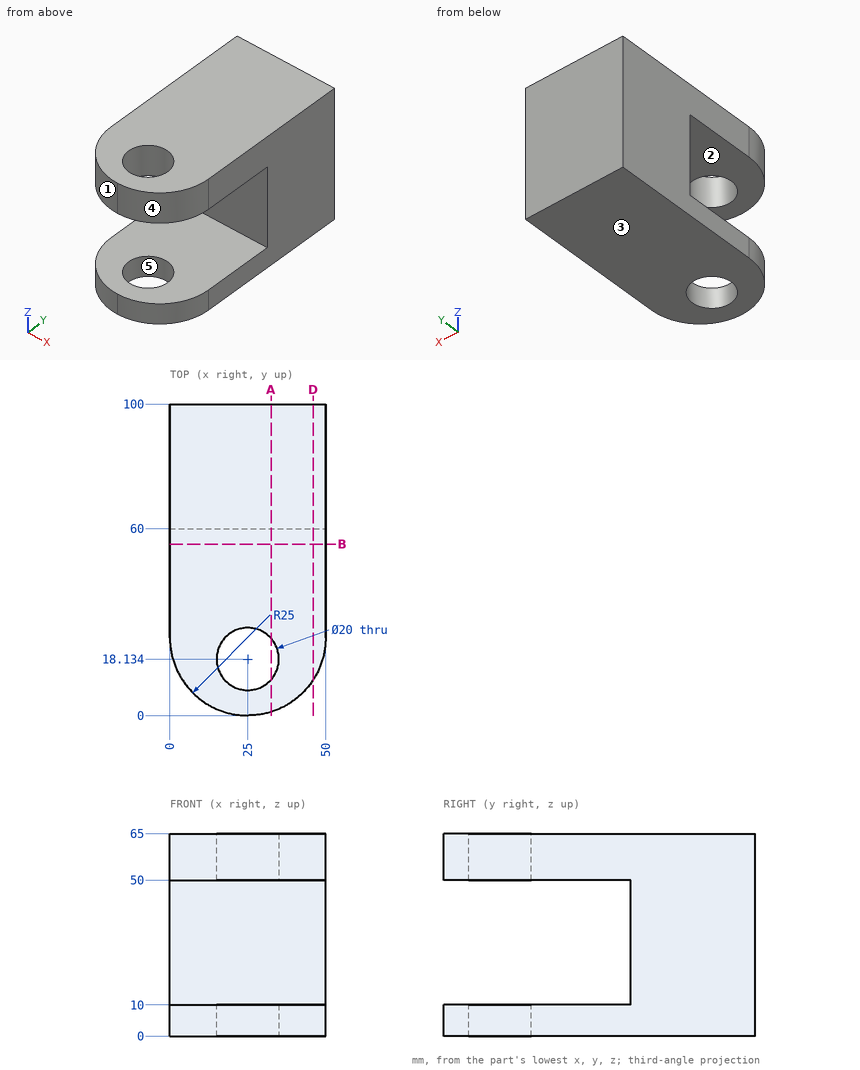
Source: three-view drawing plus pictorial views. Frame: mm from the lowest corner of the part. A direction names the side the tool comes from. Give positions to 0.01 mm unless a question says otherwise; leave off trailing zeros. Loops run counter-clockwise (first coordinate to the right, second up) from the corner with the lowest first, then second, coordinate; pieces in that order, holes last. Notation, with made-up numbers: (42, 21.25) -> (54, 21.25) arc R17 cw to (54, 30.25) -> close; hole circle Ø3 at (-8.75, -26.75). An arc over 180 degrees is marked (long way). Put each result on its own line as item: value. Start each with the question number.
1) Cut plane D-D (x = 46). Return loops of the section in (y, z) (1 decimal).
2) Contact query for flat-ended pins moving along their axis: P1, Ø5, axis at y = 16.5, z = 53, coming from the +X side; P2, Ø12, axis at x = 17, z = 21.5, coming from the -Y side. Output: stop coordinate, or through.
3) Cut plane A-A (x = 32.5). Return loops of the section in (y, z), then the cut area to 3 significant figures.
4) Cut plane B-B (y = 55). Return loops of the section in (x, z).
5) Draft query along Y for the marked faces 3, 4 and 5. Return one class per face: released by +Y, released by -Y, zero draft, split by the parting line, or undercut.
6) Material intervals for probe 1 along Z at (x, y) = (20.5, 59); probe 2 along Y at (x, z) = (25, 4); probe 3 along Y at (x, z) = (33.5, 18.5), sorted ascending.
7) Reachability of the marked faces 1 and 2 from +Z, -Z, +X, -X, +Y, -Y: full face, straight path, thin tool, end or side. Return the list, or none.
Results are:
1. outline: (11.4, 0) -> (100, 0) -> (100, 65) -> (11.4, 65) -> (11.4, 50) -> (60, 50) -> (60, 10) -> (11.4, 10) -> close
2. P1: stops at x = 49.27
2. P2: stops at y = 60
3. outline: (1.15, 0) -> (11.52, 0) -> (11.52, 10) -> (1.15, 10) -> close; (1.15, 50) -> (11.52, 50) -> (11.52, 65) -> (1.15, 65) -> close; (24.75, 0) -> (100, 0) -> (100, 65) -> (24.75, 65) -> (24.75, 50) -> (60, 50) -> (60, 10) -> (24.75, 10) -> close
3. area: 3,740 mm2
4. outline: (0, 0) -> (50, 0) -> (50, 10) -> (0, 10) -> close; (0, 50) -> (50, 50) -> (50, 65) -> (0, 65) -> close
5. face 3: zero draft
5. face 4: released by -Y
5. face 5: undercut
6. probe 1: z = 0 to 10, 50 to 65
6. probe 2: y = 0 to 8.13, 28.13 to 100
6. probe 3: y = 60 to 100
7. face 1: +Z, -Z, -X, -Y
7. face 2: +X, -X, -Y
